Model file for the job. Use its own axes, mm. A direction names the side the tool comes from. Give positions to 0.01 mm unless a question says otherwise; leave off trailing zeros. Order: outer loops, then holes, each group sorted by start corner. A loop starts at its lowest first (then second) coordinate and runs counter-clockwise, first axis right, second up. Notation, with made-up numbers: (78.5, 83.25) -> (97.5, 83.25) arc R20 ccw to (97.5, 116.25) -> close; hole circle Ø9 at (22, 72). An arc over 180 degrees is marked (long way). Answer in a Markdown table with one row per item. Add a question column.
from build123d import *

# Parameters (mm, degrees)
F0_W     = 36.73077
F0_H     = 18.46154
F1_DEPTH = 11.8
F2_R     = 2.124108
F3_DEPTH = 25
F4_W     = 24.038464
F4_H     = 6.153846
F5_DEPTH = 4.6


with BuildPart() as f1:
    # F0 (on Front) → F1 (new body)
    with BuildSketch(Plane.XZ):
        with Locations((0.096153, 0.288462)):
            Rectangle(F0_W, F0_H)
    extrude(amount=F1_DEPTH)

    # F2 (on Front) → F3 (join)
    with BuildSketch(Plane.XZ):
        with Locations((-12.884616, -4.711539)):
            Circle(F2_R)
    extrude(amount=F3_DEPTH)

    # F4 (on Front) → F5 (cut)
    with BuildSketch(Plane.XZ):
        with Locations((-12.019232, -5.096154)):
            Rectangle(F4_W, F4_H)
    extrude(amount=F5_DEPTH, mode=Mode.SUBTRACT)


solid = f1.part
Item 1: Saw through at D-D on z = 6.25. List the corners of the cut face in (x, y).
Item 2: Wall check: line 1 (Y direction, x = 1, z = -3.5); line 2 (Y direction, x = -3, z = -5.75); line 3 (X direction, y = -12, z = -4). Give the ranges that are in metal, low to high.
Item 3: Saw through at A-A on x = -7. List the corners of the cut face in (y, z).
Item 4: Saw through at B-B on y = -2.5. List the corners of the cut face in (x, z).
Item 5: Pin check, flat tips, straight feed: pin 1 Ø3 at (x, z) = (-12, -6) entering from +Y; pin 2 Ø6 at (x, z) = (-11, -2) entering from -Y; pin 3 Ø2 at (x, z) = (-2.5, 5.5) entering from -Y; pin 4 Ø2.5 at (y, z) = (-3, -4) entering from -X. Stop position of each tip, or through.
Item 6: Two-plate mould, pull along Z, no slides. Class faces 4 (the flat face through (0, -2, -5)), 5 (the flat face through (-13, -25, -5)), 6 (the flat face through (0, -6, 9.519)): pulls with the +Z half, pulls with the -Z half, needs draft (parallel to the pull), parting line crosses it, or undercut.
Item 7: Which spindle directions (+Z, -Z, +X, -X, +Y, -Y) get a long thin tool onto all of the face, cutting with end or side? Do faces 1 (the cylindrical face through (-11.74, -18.31, -2.92)), 2 (the flat face through (-9, -4.6, -5)), 3 (the flat face through (0, -6, -8.942)). Say none if no direction does.
Item 8: Saw through at C-C on z = -5.25. List the corners of the cut face in (x, y).
Evaluation:
| question | item | result |
|---|---|---|
| 1 | outline | (-18.27, -11.8) -> (18.46, -11.8) -> (18.46, 0) -> (-18.27, 0) -> close |
| 2 | line 1 | y = -11.8 to 0 |
| 2 | line 2 | y = -11.8 to -4.6 |
| 2 | line 3 | x = -14.89 to -10.88 |
| 3 | outline | (-11.8, -8.94) -> (0, -8.94) -> (0, -8.17) -> (-4.6, -8.17) -> (-4.6, -2.02) -> (0, -2.02) -> (0, 9.52) -> (-11.8, 9.52) -> close |
| 4 | outline | (-18.27, -8.94) -> (18.46, -8.94) -> (18.46, 9.52) -> (-18.27, 9.52) -> (-18.27, -2.02) -> (0, -2.02) -> (0, -8.17) -> (-18.27, -8.17) -> close |
| 5 | pin 1 | stops at y = -4.6 |
| 5 | pin 2 | stops at y = -25 |
| 5 | pin 3 | stops at y = -11.8 |
| 5 | pin 4 | stops at x = 0 |
| 6 | face 4 | undercut |
| 6 | face 5 | needs draft |
| 6 | face 6 | pulls with the +Z half |
| 7 | face 1 | -Y |
| 7 | face 2 | -X, +Y |
| 7 | face 3 | -Z, +X, -X, +Y, -Y |
| 8 | outline | (-18.27, -11.8) -> (-14.94, -11.8) -> (-14.94, -25) -> (-10.83, -25) -> (-10.83, -11.8) -> (18.46, -11.8) -> (18.46, 0) -> (0, 0) -> (0, -4.6) -> (-18.27, -4.6) -> close |
